Part print with two shaded views. Sizes in mm from the minimum x, y, z corner. A direction names the side the tool comes from. Round coordinates to 2 decimals unless told otherwise and drop trailing zeros. Loops run counter-clockwise (first coordinate to the right, second up) from the corner with the lowest first, then second, coordinate; pieces in that order, holes last. Notation, with made-up numbers: (36, 12) - (81, 12) arc R22 cw to (81, 42) - close; hole circle Ø4 at (-18, -24). An arc over 180 degrees is marked (long way). Use a Markdown table: item, result.
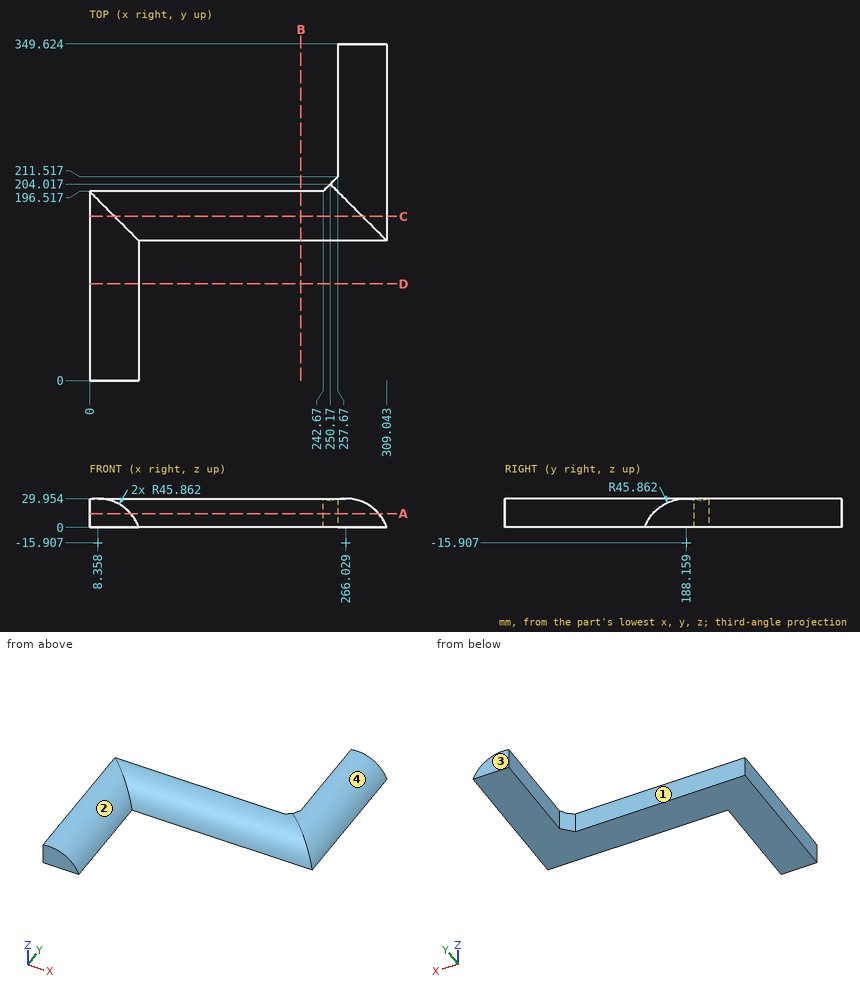
Q1. Cut at C-C, the plane y = 170.5. List the corners of the cut face in (x, z).
Results found:
| item | result |
|---|---|
| outline | (0, 0) - (309.04, 0) arc R45.86 ccw to (283.69, 26.42) - (26.02, 26.42) arc R45.86 ccw to (0, 29.19) - close |
Q2. Probe line 1 (X direction, y = 234, z = 15); line 2 (X direction, y = 177, z = 13.5); line 3 (Y direction, x = 87, z = 18.75) (1 decimal). List the from-to ranges inside material, lowest first.
Results found:
| item | result |
|---|---|
| line 1 | x = 257.67 to 299.91 |
| line 2 | x = 0 to 301.22 |
| line 3 | y = 158.1 to 196.5 |
Q3. Which spindle directions (+Z, -Z, +X, -X, +Y, -Y) get a long thin tool onto all of the face, cutting with end or side? Do the marked faces 1, 2, 3 and 4. Say none if no direction does.
Results found:
| item | result |
|---|---|
| face 1 | +Z, -Z, -X, +Y |
| face 2 | +Z, -Y |
| face 3 | +Z, -Z, +X, -X, +Y |
| face 4 | +Z, +Y |
Q4. Cut at D-D, the plane y = 100.5. List the corners of the cut face in (x, z), plus the area to 3 significant figures.
Results found:
| item | result |
|---|---|
| outline | (0, 0) - (51.37, 0) arc R45.86 ccw to (0, 29.19) - close |
| area | 1,190 mm2 |
Q5. Cut at A-A, the plane z = 14.25. List the corners of the cut face in (x, y).
Results found:
| item | result |
|---|---|
| outline | (0, 0) - (42.91, 0) - (42.91, 153.61) - (300.58, 153.61) - (300.58, 349.62) - (257.67, 349.62) - (257.67, 211.52) - (242.67, 196.52) - (0, 196.52) - close |
Q6. Drop flat-ended pins along their axis: pin 1 (3 mm diameter, centred on y = 239, z = 20, fed in from +X); pin 2 (5 mm diameter, centred on x = 268, z = 6, fed in from -Y) (1 decimal); pin 3 (5 mm diameter, centred on x = 174.5, z = 3.5, fed in from +Y). Give the stop position or say it passes through.
Results found:
| item | result |
|---|---|
| pin 1 | stops at x = 296.35 |
| pin 2 | stops at y = 146.6 |
| pin 3 | stops at y = 196.52 |
Q7. Cut at B-B, the plane x = 219.5. List the corners of the cut face in (y, z) (1 decimal), plus the area to 3 significant figures.
Results found:
| item | result |
|---|---|
| outline | (145.1, 0) - (196.5, 0) - (196.5, 29.2) arc R45.9 ccw to start |
| area | 1,190 mm2 |
